Source: CAD feature listing. Evaluate the final solid. Frame: model axes, mm. A direction names the side the tool comes from. Coordinates: 2 decimals unless noted, no trailing zeros. Loops run counter-clockwise (first coordinate to the right, second up) from the corner with the lowest first, then second, coordinate; pieces in that order, holes last. Notation, with made-up numbers: M -19.5,36.5 L 25.5,36.5 A22 cw 25.5,67.5 Z; hole C 42,50.5 d7. An arc over 180 degrees is marked long. Write each question's results on one line, items separated by ' | '. Start each with the question number.
from build123d import *

# Parameters (mm, degrees)
SKETCH1_R                = 1.5875
BOSS_EXTRUDE1_DEPTH      = 2.54
BOSS_EXTRUDE2_DEPTH      = 11.43
BOSS_EXTRUDE2_DEPTH_BACK = 2.54
SKETCH2_W                = 44.45
SKETCH2_H                = 3.175
SKETCH3_R                = 2.413
CUT_EXTRUDE1_DEPTH       = 33.139163755
FILLET1_R                = 6.35


with BuildPart() as part:
    # Sketch1 → Boss-Extrude1 (new body)
    with BuildSketch(Plane.XY):
        with BuildLine():
            Line((-8.255, -5.230769231), (-8.255, 0.738461538))
            Line((-8.255, 0.738461538), (-16.6624, 0.738461538))
            Line((-16.6624, 0.738461538), (-16.6624, -5.230769231))
            Line((-16.6624, -5.230769231), (-16.6624, -20.978769231))
            Line((-16.6624, -20.978769231), (16.6624, -20.978769231))
            Line((16.6624, -20.978769231), (16.6624, -5.230769231))
            Line((16.6624, -5.230769231), (16.6624, 0.738461538))
            Line((16.6624, 0.738461538), (8.255, 0.738461538))
            Line((8.255, 0.738461538), (8.255, -5.230769231))
            ThreePointArc((8.255, -5.230769231), (0, -13.485769231), (-8.255, -5.230769231))
        make_face()
        with Locations((-12.4587, -5.230769231)):
            Circle(SKETCH1_R, mode=Mode.SUBTRACT)
        with Locations(Location((12.4587, -5.230769231, 0), (0, 0, 180))):
            Circle(SKETCH1_R, mode=Mode.SUBTRACT)
    extrude(amount=BOSS_EXTRUDE1_DEPTH)

    # Sketch2 → Boss-Extrude2 (add, two sides: drawn at the far end of the back side and taken through both)
    with BuildSketch(Plane.XY.offset(2.54).offset(-BOSS_EXTRUDE2_DEPTH_BACK)):
        with Locations((0, -19.391269231)):
            Rectangle(SKETCH2_W, SKETCH2_H)
    extrude(amount=BOSS_EXTRUDE2_DEPTH + BOSS_EXTRUDE2_DEPTH_BACK)

    # Sketch3 → Cut-Extrude1 (cut, through all)
    with BuildSketch(Plane(origin=(0, -17.803769231, 0), x_dir=(1, 0, 0), z_dir=(0, 1, 0))):
        with Locations(Location((-16.51, -8.255, 0), (0, 0, 270))):
            Circle(SKETCH3_R)
        with Locations(Location((16.51, -8.255, 0), (0, 0, 90))):
            Circle(SKETCH3_R)
    extrude(amount=-CUT_EXTRUDE1_DEPTH, mode=Mode.SUBTRACT)

    # Fillet1
    # the kernel refuses this fillet: 6.35 mm, written as the material it adds along each edge
    with BuildSketch(Plane(origin=(-16.6624, -17.803769231, 2.54), x_dir=(0, 1, 0), z_dir=(0, 0, -1))) as fillet1_piece_1:
        with BuildLine():
            CenterArc((6.300992084, -6.35), FILLET1_R, 90, 82.87698928)
            Line((0, -5.5626), (-0.126019842, -5.546852))
            ThreePointArc((-0.126019842, -5.546852), (-0.127, -2.7813), (-0.127, 0))
            Line((-0.127, 0), (0, 0.127))
            Line((0, 0.127), (6.300992084, 0.127))
            Line((6.300992084, 0.127), (6.300992084, 0))
        make_face()
    extrude(amount=2.54)
    with BuildSketch(Plane(origin=(16.6624, -17.803769231, 0), x_dir=(1, 0, 0), z_dir=(0, 0, 1))) as fillet1_piece_2:
        with BuildLine():
            CenterArc((6.35, 6.300992084), FILLET1_R, 180, 82.87698928)
            Line((0, 6.300992084), (-0.127, 6.300992084))
            Line((-0.127, 6.300992084), (-0.127, 0))
            Line((-0.127, 0), (0, -0.127))
            ThreePointArc((0, -0.127), (2.7813, -0.127), (5.546852, -0.126019842))
            Line((5.546852, -0.126019842), (5.5626, 0))
        make_face()
    extrude(amount=2.54)


solid = part.part
Item 1: Cut plane B-B (y = -11). Output: boundary loops of the cut face in (x, z).
Item 2: Line query: probe 1 along Z at (x, y) = (16.51, -19.95); probe 2 along X at (y, z) = (-18.5, 7.25) (3 decimals); probe 3 along Y at (x, z) = (-5.5, 7.5). Output: solid intervals per line, ascending.
Item 3: Mould query, pull axis X, two halves, no side actions, for faces 6 (the flat face through (13, 0.738, 1)), 7 (the cylindrical face through (0.182, -13.484, 1.252)), 8 (the flat face through (-22.225, -19, 7)). Classes: +X half, -X half, draft (parallel to the pull), parting line (faces both ways), or undercut.
Item 4: First-contact query: pin 1 Ø3.5 at (x, y) = (-12.46, -5.23) entering from +Z; pin 2 Ø3 at (y, z) = (-4, 1) entering from +X; pin 3 Ø1.5 at (x, z) = (-17, 10) entering from +Y; pin 4 Ø6 at (y, z) = (-10.5, 6.5) entering from -X. Flat tips, straight axial feed; report the tip coordinate or a pass-through.
Item 5: Cut plane D-D (z = 6.5). Output: boundary loops of the cut face in (x, y) (3 decimals).
Item 6: Access query for faces 1 (the flat face through (0, -19, 13.97)), 2 (the flat face through (0, -17.804, 8)), 3 (the flat face through (16.662, -5, 1)), 4 (the flat face through (-16.662, -5, 1)), 5 (the flat face through (-8.255, -2, 1)). Directions: +Z, -Z, +X, -X, +Y, -Y. A direction counts if a zero-diameter tool reaches every point of the face in a straight line with its end or side. Return the directions, or none.
Item 7: Cut plane C-C (x = 16). Output: boundary loops of the cut face in (y, z), then the cut area to 3 significant figures.
Item 8: Cut plane A-A (z = 1). Count the separate pieces of the cut face and the enclosed holes in it, then the cut area to 3 significant figures.
Response values:
1) outline: M -16.66,0 L -5.9,0 L -5.9,2.54 L -16.66,2.54 Z; M 5.9,0 L 16.66,0 L 16.66,2.54 L 5.9,2.54 Z
2) probe 1: z = 0 to 5.84, 10.67 to 13.97 | probe 2: x = -22.225 to -18.704, -14.316 to 14.316, 18.704 to 22.225 | probe 3: y = -20.98 to -17.8
3) face 6: draft | face 7: undercut | face 8: -X half
4) pin 1: stops at z = 2.54 | pin 2: stops at x = 16.66 | pin 3: stops at y = -17.8 | pin 4: passes through
5) outline: M -22.225,-20.979 L -18.166,-20.979 L -18.166,-17.804 L -22.225,-17.804 Z; M -14.854,-20.979 L 14.854,-20.979 L 14.854,-17.804 L -14.854,-17.804 Z; M 18.166,-20.979 L 22.225,-20.979 L 22.225,-17.804 L 18.166,-17.804 Z
6) face 1: +Z, +X, -X, +Y, -Y | face 2: +Z, +X, -X, +Y | face 3: +Z, -Z, +X, +Y | face 4: +Z, -Z, -X, +Y | face 5: +Z, -Z, +Y
7) outline: M -20.98,0 L 0.74,0 L 0.74,2.54 L -17.8,2.54 L -17.8,5.9 L -20.98,5.9 Z; M -20.98,10.61 L -17.8,10.61 L -17.8,13.97 L -20.98,13.97 Z | area: 76.5 mm2
8) separate pieces: 1 | enclosed holes: 2 | area: 554 mm2
